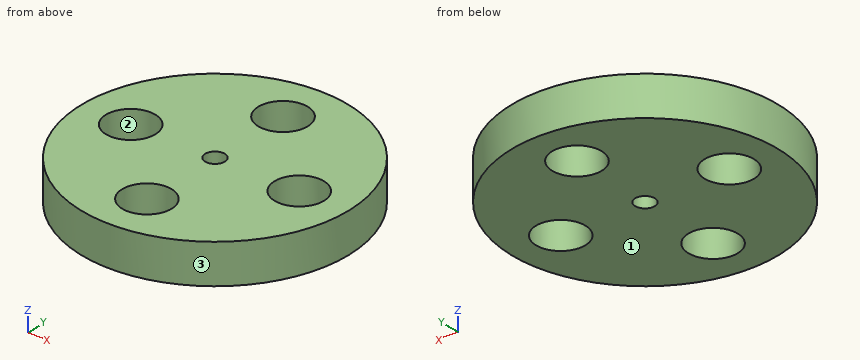
from build123d import *

# Parameters (mm, degrees)
SKETCH1_R           = 13.5
BOSS_EXTRUDE1_DEPTH = 4
CUT_EXTRUDE1_REACH  = 21.506
SKETCH2_R           = 1
CUT_EXTRUDE2_REACH  = 21.506
SKETCH3_R           = 2.5
CUT_EXTRUDE3_REACH  = 21.506
SKETCH4_R           = 2.5
CUT_EXTRUDE4_REACH  = 21.506
SKETCH5_R           = 2.5


with BuildPart() as part:
    # Sketch1 → Boss-Extrude1 (new body)
    with BuildSketch(Plane.XY):
        Circle(SKETCH1_R)
    extrude(amount=BOSS_EXTRUDE1_DEPTH)

    # Sketch2 → Cut-Extrude1 (cut, up to next)
    with BuildSketch(Plane.XY.offset(4), mode=Mode.PRIVATE) as cut_extrude1_sk1:
        Circle(SKETCH2_R)
    cut_extrude1_tool1 = extrude(cut_extrude1_sk1.sketch, amount=-CUT_EXTRUDE1_REACH, mode=Mode.PRIVATE) & part.part
    add(cut_extrude1_tool1.solids().sort_by_distance((0, 0, 4))[0], mode=Mode.SUBTRACT)

    # Sketch3 → Cut-Extrude2 (cut, up to next)
    with BuildSketch(Plane(origin=(0, 0, 0), x_dir=(-1, 0, 0), z_dir=(0, 0, -1)), mode=Mode.PRIVATE) as cut_extrude2_sk1:
        with Locations((0, 8.5)):
            Circle(SKETCH3_R)
    cut_extrude2_tool1 = extrude(cut_extrude2_sk1.sketch, amount=-CUT_EXTRUDE2_REACH, mode=Mode.PRIVATE) & part.part
    cut_extrude2 = cut_extrude2_tool1.solids().sort_by_distance((0, 8.5, 0))[0]
    add(cut_extrude2, mode=Mode.SUBTRACT)

    # Mirror1: Cut-Extrude2 across plane
    add(cut_extrude2.mirror(Plane.ZX), mode=Mode.SUBTRACT)

    # Sketch4 → Cut-Extrude3 (cut, up to next)
    with BuildSketch(Plane(origin=(0, 0, 0), x_dir=(-1, 0, 0), z_dir=(0, 0, -1)), mode=Mode.PRIVATE) as cut_extrude3_sk1:
        with Locations((8.5, 0)):
            Circle(SKETCH4_R)
    cut_extrude3_tool1 = extrude(cut_extrude3_sk1.sketch, amount=-CUT_EXTRUDE3_REACH, mode=Mode.PRIVATE) & part.part
    add(cut_extrude3_tool1.solids().sort_by_distance((-8.5, 0, 0))[0], mode=Mode.SUBTRACT)

    # Sketch5 → Cut-Extrude4 (cut, up to next)
    with BuildSketch(Plane(origin=(0, 0, 0), x_dir=(-1, 0, 0), z_dir=(0, 0, -1)), mode=Mode.PRIVATE) as cut_extrude4_sk1:
        with Locations((-8.5, 0)):
            Circle(SKETCH5_R)
    cut_extrude4_tool1 = extrude(cut_extrude4_sk1.sketch, amount=-CUT_EXTRUDE4_REACH, mode=Mode.PRIVATE) & part.part
    add(cut_extrude4_tool1.solids().sort_by_distance((8.5, 0, 0))[0], mode=Mode.SUBTRACT)


solid = part.part
Read the model definition and answer for the solid it produces. Units are mm, in the model's axes. Face numbers are marked on the shaded views. Coordinates: 2 decimals unless noted, no trailing zeros. Write each loop counter-clockwise with the first axis right and the second up, starting at its lowest first coordinate (ties: lowest second). Pieces come first, ordered by that corner, then holes. Notation, with made-up numbers: M 88.5,-0.75 L 97.5,-0.75 A10 ccw 97.5,11.25 Z; hole C 20,66.25 d9. An arc over 180 degrees is marked long. Use a Markdown table: item, result.
Q1. The part is cut by section A-A, the plane y = 0. Write down the section's boundary in (x, z), then the cut area to 3 significant figures.
Answer block:
| item | result |
|---|---|
| outline | M -13.5,0 L -11,0 L -11,4 L -13.5,4 Z; M -6,0 L -1,0 L -1,4 L -6,4 Z; M 1,0 L 6,0 L 6,4 L 1,4 Z; M 11,0 L 13.5,0 L 13.5,4 L 11,4 Z |
| area | 60.0 mm2 |
Q2. Determine the mould class of the marked faces 1, 2 and 3 for opening direction Y: released by +Y, released by -Y, zero draft, split by the parting line, or undercut.
Answer block:
| item | result |
|---|---|
| face 1 | zero draft |
| face 2 | undercut |
| face 3 | split by the parting line |
Q3. The part is cut by section D-D, the plane x = 6.5. Write down the section's boundary in (y, z), then the cut area to 3 significant figures.
Answer block:
| item | result |
|---|---|
| outline | M -11.83,0 L -1.5,0 L -1.5,4 L -11.83,4 Z; M 1.5,0 L 11.83,0 L 11.83,4 L 1.5,4 Z |
| area | 82.7 mm2 |
Q4. The part is cut by section C-C, the plane z = 1.35. Write down the section's boundary in (x, y), then the cut area to 3 significant figures.
Answer block:
| item | result |
|---|---|
| outline | C 0,0 d27; hole C -8.5,0 d5; hole C 0,-8.5 d5; hole C 0,8.5 d5; hole C 0,0 d2; hole C 8.5,0 d5 |
| area | 491 mm2 |
Q5. Each of these flat-tipped pins is pushed along its axis until it touches: pin 1 Ø3 at (x, y) = (8.5, 0) entering from -Z; pin 2 Ø1.5 at (y, z) = (-3, 1.5) entering from +X. Where does it stop, or does it pass through?
Answer block:
| item | result |
|---|---|
| pin 1 | passes through |
| pin 2 | stops at x = 13.31 |
Q6. Straight lines are drawn through the part: L1, parallel to Y at x = 0, z = 1.3; L2, parallel to Y at x = -2, z = 1.4; L3, parallel to X at y = 0.25, z = 0.4. For each, find the intervals that lie inside material, in ascending order. Write a range as [from, to].
Answer block:
| item | result |
|---|---|
| L1 | y = [-13.5, -11], [-6, -1], [1, 6], [11, 13.5] |
| L2 | y = [-13.35, -10], [-7, 7], [10, 13.35] |
| L3 | x = [-13.5, -10.99], [-6.01, -0.97], [0.97, 6.01], [10.99, 13.5] |
